from build123d import *

# Parameters (mm, degrees)
F0_W         = 124.0848004818
F0_H         = 75.9339258075
F1_DEPTH     = 3.6583524197
F2_R         = 5.08
F3_T1_DEPTH  = 113.9248004818
F3_T3_DEPTH  = 65.7739258075
F3_T6_ANGLE  = 90
F3_T8_ANGLE  = 90
F3_T10_ANGLE = 90
F3_T12_ANGLE = 90


# Not quite as in the source:
# - a fillet or chamfer that OpenCascade refuses, or shapes differently, is made with other operations: its cross-section is extruded or revolved along the edge and cut away or added


with BuildPart() as f1:
    # F0 (on Top) → F1 (new body)
    with BuildSketch(Plane.XY):
        with Locations((-32.2462767363, 8.972465992)):
            Rectangle(F0_W, F0_H)
    extrude(amount=-F1_DEPTH)

    # F2
    f2_edges = [f1.edges().sort_by_distance(p)[0] for p in [
        (29.796124, 46.939429, -1.829176),
        (29.796124, -28.994497, -1.829176),
        (-94.288677, 46.939429, -1.829176),
        (-94.288677, -28.994497, -1.829176),
    ]]
    fillet(f2_edges, radius=F2_R)

    # F3: fillet of radius 5.08 on 1 edges, made by hand

    # F3_s2 → F3_t1 (cut)
    with BuildSketch(Plane.YZ.offset(-89.2086769772)):
        with BuildLine():
            ThreePointArc((42.0624095029, 0), (45.110722995, -1.016235138), (46.9394288957, -3.6583524197))
            Line((46.9394288957, -3.6583524197), (46.9394288957, 0))
            Line((46.9394288957, 0), (42.0624095029, 0))
        make_face()
        with BuildLine():
            ThreePointArc((-24.117477519, 0), (-27.1657910111, -1.016235138), (-28.9944969118, -3.6583524197))
            Line((-28.9944969118, -3.6583524197), (-28.9944969118, 0))
            Line((-28.9944969118, 0), (-24.117477519, 0))
        make_face()
    extrude(amount=F3_T1_DEPTH, mode=Mode.SUBTRACT)

    # F3_s4 → F3_t3 (cut)
    with BuildSketch(Plane.XZ.offset(-41.8594288957)):
        with BuildLine():
            ThreePointArc((-89.4116575844, 0), (-92.4599710765, -1.016235138), (-94.2886769772, -3.6583524197))
            Line((-94.2886769772, -3.6583524197), (-94.2886769772, 0))
            Line((-94.2886769772, 0), (-89.4116575844, 0))
        make_face()
        with BuildLine():
            ThreePointArc((29.7961235046, -3.6583524197), (27.967417604, -1.016235138), (24.9191041119, 0))
            Line((24.9191041119, 0), (29.7961235046, 0))
            Line((29.7961235046, 0), (29.7961235046, -3.6583524197))
        make_face()
    extrude(amount=F3_T3_DEPTH, mode=Mode.SUBTRACT)

    # F3_s5 → F3_t6 (revolve, cut)
    with BuildSketch(Plane.YZ.offset(-89.2086769772)):
        with BuildLine():
            ThreePointArc((42.0624095029, 0), (45.110722995, -1.016235138), (46.9394288957, -3.6583524197))
            Line((46.9394288957, -3.6583524197), (46.9394288957, 0))
            Line((46.9394288957, 0), (42.0624095029, 0))
        make_face()
    revolve(axis=Axis((-89.2086769772, 41.8594288957, 0), (0, 0, 1)), revolution_arc=F3_T6_ANGLE, mode=Mode.SUBTRACT)

    # F3_s7 → F3_t8 (revolve, cut)
    with BuildSketch(Plane.XZ.offset(23.9144969118)):
        with BuildLine():
            ThreePointArc((-89.4116575844, 0), (-92.4599710765, -1.016235138), (-94.2886769772, -3.6583524197))
            Line((-94.2886769772, -3.6583524197), (-94.2886769772, 0))
            Line((-94.2886769772, 0), (-89.4116575844, 0))
        make_face()
    revolve(axis=Axis((-89.2086769772, -23.9144969118, 0), (0, 0, 1)), revolution_arc=F3_T8_ANGLE, mode=Mode.SUBTRACT)

    # F3_s9 → F3_t10 (revolve, cut)
    with BuildSketch(Plane.XZ.offset(23.9144969118)):
        with BuildLine():
            ThreePointArc((24.9191041119, 0), (27.967417604, -1.016235138), (29.7961235046, -3.6583524197))
            Line((29.7961235046, -3.6583524197), (29.7961235046, 0))
            Line((29.7961235046, 0), (24.9191041119, 0))
        make_face()
    revolve(axis=Axis((24.7161235046, -23.9144969118, 0), (0, 0, -1)), revolution_arc=F3_T10_ANGLE, mode=Mode.SUBTRACT)

    # F3_s11 → F3_t12 (revolve, cut)
    with BuildSketch(Plane.XZ.offset(-41.8594288957)):
        with BuildLine():
            ThreePointArc((24.9191041119, 0), (27.967417604, -1.016235138), (29.7961235046, -3.6583524197))
            Line((29.7961235046, -3.6583524197), (29.7961235046, 0))
            Line((29.7961235046, 0), (24.9191041119, 0))
        make_face()
    revolve(axis=Axis((24.7161235046, 41.8594288957, 0), (0, 0, 1)), revolution_arc=F3_T12_ANGLE, mode=Mode.SUBTRACT)


solid = f1.part
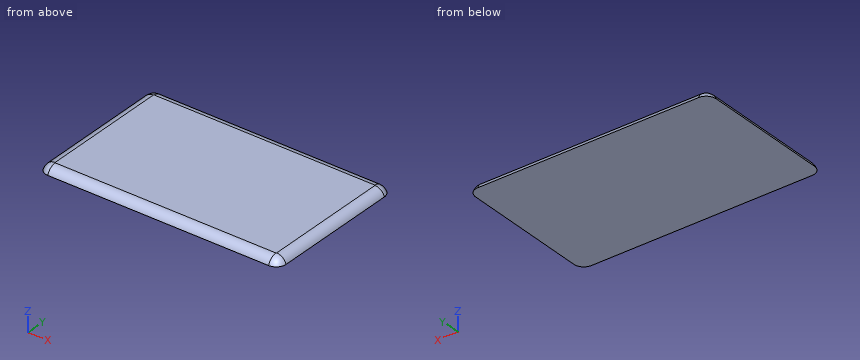
Check sheet for the modelled part. Datum: model origin and axes. Units: mm. Give positions to 0.01 mm unless a question says otherwise; leave off trailing zeros. Write each loop counter-clockwise with the first axis right and the second up, starting at its lowest first coordinate (ties: lowest second). Pieces come first, ordered by that corner, then holes. Notation, with made-up numbers: (45, 35) -> (69, 35) arc R18 cw to (69, 59) -> close; hole circle Ø5 at (9.25, 11). An arc over 180 degrees is marked (long way). Write item = value, one per line.
Item 1: Gauge pin test, flat ends, axial feed: pin 1 (2 mm diameter, centred on y = -6.5, z = -0.5, fed in from -X); pin 2 (1 mm diameter, centred on x = -17.5, z = -1.5, fed in from +Y); pin 3 (2 mm diameter, centred on y = 29, z = -2.5, fed in from -X). Record the tip position at first contact, or that the pin passes through.
Output:
pin_1 = -93.02
pin_2 = 46.1
pin_3 = -94.24
Item 2: Scan lines: probe 1 along X at (y, z) = (-18, -0.5); probe 2 along X at (y, z) = (-7.5, -1.05); probe 3 along Y at (x, z) = (-53, -1.35). Record each from-to range of solid material in increasing order. Write a range as from..to.
Output:
probe_1 = -91.61..27.12
probe_2 = -92.5..28.01
probe_3 = -27.57..45.51
Item 3: Sectioned sample at A-A on y = -15.5. Record the boundary of the cut face in (x, z), and give its area (3 significant figures).
Output:
outline = (-94.29, -3.66) -> (29.8, -3.66) arc R5.08 ccw to (24.92, 0) -> (-89.41, 0) arc R5.08 ccw to start
area = 445 mm^2
Item 4: Sectioned sample at B-B on x = -7. Record the boundary of the cut face in (y, z).
Output:
outline = (-28.99, -3.66) -> (46.94, -3.66) arc R5.08 ccw to (42.06, 0) -> (-24.12, 0) arc R5.08 ccw to start
